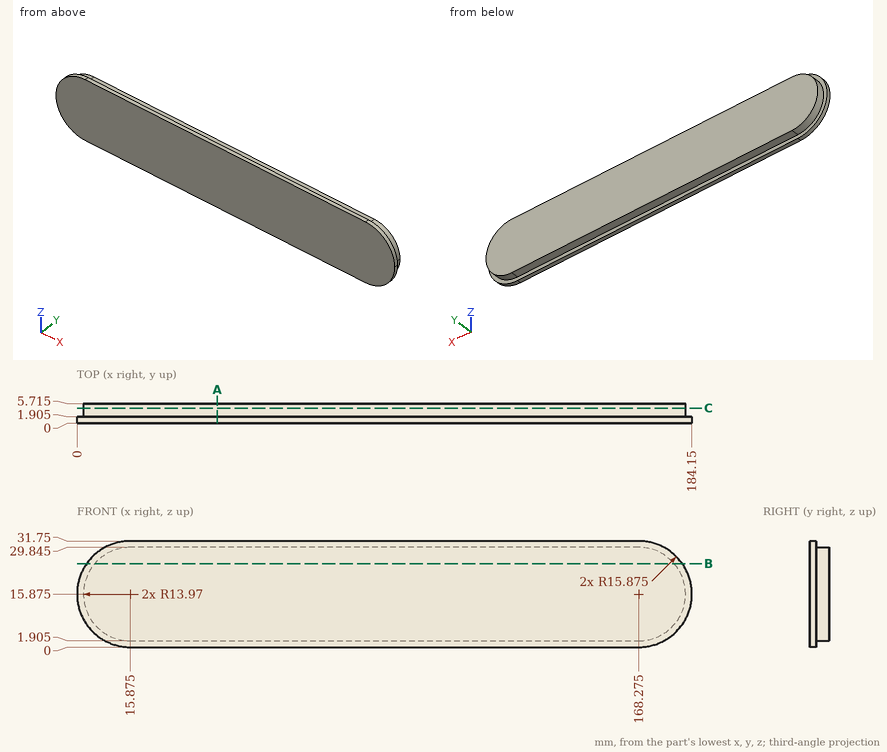
Can you work these out from the drawing? Everything is in mm from the part's minimum corner. Give positions to 0.01 mm unless a question says otherwise; leave off trailing zeros. Order: outer loops, then holes, each group sorted by start corner. A loop starts at its lowest first (then second) coordinate and runs counter-clockwise, first axis right, second up.
Item 1: If we section it at A-A, the plane x = 42: Write out the boundary of the cut face in (y, z) (3 decimals).
Item 2: If we section it at C-C, the plane y = 4.5: Write out the boundary of the cut face in (x, z) (3 decimals), plus the area to 3 significant figures.
Item 3: I'm going to push flat-ended pins straight in: pin 1 (1.9 mm diameter, centred on x = 62, y = 3.5, fed in from +Z) (3 decimals); pin 2 (3 mm diameter, centred on y = 1.5, z = 21, fed in from +X); pin 3 (4 mm diameter, centred on x = 81, z = 16.5, fed in from -Y). Where does each tip first touch, or does it pass through?
Item 4: I need wall thicknesses on line 1 (Z direction, x = 101.5, y = 4.3) (3 decimals); line 2 (X direction, y = 3.2, z = 16); line 3 (X direction, y = 4.85, z = 19). Which ranges of each line are inside material? Lowest first, please.
Item 5: If we section it at B-B, the plane z = 25: Write out the boundary of the cut face in (x, y) (3 decimals).
Values:
1. outline: (0, 0) - (1.905, 0) - (1.905, 1.905) - (5.715, 1.905) - (5.715, 29.845) - (1.905, 29.845) - (1.905, 31.75) - (0, 31.75) - close
2. outline: (15.875, 1.905) - (168.275, 1.905) arc R13.97 ccw to (168.275, 29.845) - (15.875, 29.845) arc R13.97 ccw to start
2. area: 4,870 mm2
3. pin 1: stops at z = 29.845
3. pin 2: stops at x = 183.73
3. pin 3: stops at y = 0
4. line 1: z = 1.905 to 29.845
4. line 2: x = 1.91 to 182.24
4. line 3: x = 2.26 to 181.89
5. outline: (2.885, 0) - (181.265, 0) - (181.265, 1.905) - (178.853, 1.905) - (178.853, 5.715) - (5.297, 5.715) - (5.297, 1.905) - (2.885, 1.905) - close
